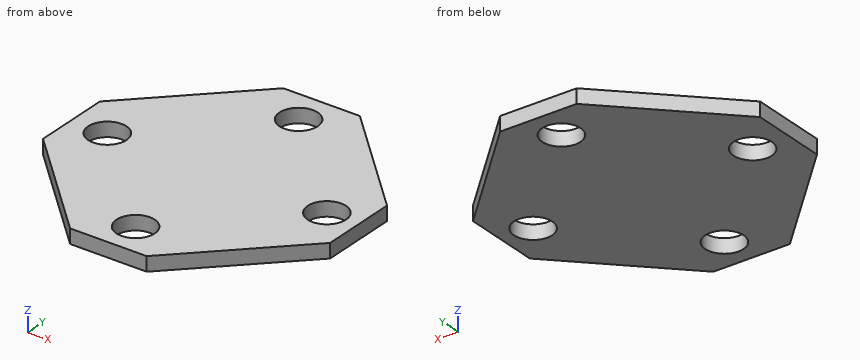
from build123d import *

# Parameters (mm, degrees)
BOSS_EXTRUDE2_DEPTH = 3
SKETCH1_3_R         = 4
CUT_EXTRUDE1_DEPTH  = 4
CIRPATTERN4_COUNT   = 4


with BuildPart() as part:
    # Sketch1 → Boss-Extrude2 (new body)
    with BuildSketch(Plane.XY):
        Polygon((-8, 30), (-30, 8), (-30, -8), (-8, -30), (8, -30), (30, -8), (30, 8), (8, 30), align=None)
    extrude(amount=BOSS_EXTRUDE2_DEPTH)

    # Sketch1<3> → Cut-Extrude1 (cut, through all)
    with BuildSketch(Plane.XY):
        with Locations((-22.5, 0)):
            Circle(SKETCH1_3_R)
    cut_extrude1 = extrude(amount=CUT_EXTRUDE1_DEPTH, mode=Mode.SUBTRACT)

    # CirPattern4: Cut-Extrude1 ×4 about axis
    cirpattern4_axis = Axis((0.438067256, 0, 0), (0, 0, 1))
    for i in range(1, CIRPATTERN4_COUNT):
        add(cut_extrude1.rotate(cirpattern4_axis, i * 360 / CIRPATTERN4_COUNT), mode=Mode.SUBTRACT)


solid = part.part
The listing builds one solid part. Answer for the finished solid, in the listing's coordinates (mm). Round coordinates to 2 decimals unless told otherwise and drop trailing zeros. Write each loop counter-clockwise with the first axis right and the second up, starting at its lowest first coordinate (ties: lowest second). Pieces come first, ordered by that corner, then holes. Notation, with made-up numbers: M 14.25,-24.5 L 25.25,-24.5 A20 ccw 25.25,3.5 Z; hole C -39.75,50 d1. An arc over 180 degrees is marked long. Write each question's results on one line, items separated by ' | '. Start each with the question number.
Item 1: A flat-ended cylindrical pin translates along its axis: pin 1 Ø1.5 at (x, z) = (17.5, 0.5) entering from -Y. Find the tip coordinate at first contact, or state that the pin passes through.
Item 2: A cutting plane is placed at B-B on y = 0. Write down the section's boundary in (x, z), and give its area (3 significant figures).
Item 3: A cutting plane is placed at C-C on z = 1.25. Write down the section's boundary in (x, y), and give its area (3 significant figures).
Item 4: Straight lines are drawn through the part: L1, parallel to X at y = 0, z = 2.4; L2, parallel to X at y = 3.5, z = 1.25; L3, parallel to Y at x = 0.5, z = 2.35. For each, find the intervals that lie inside material, in ascending order. Write a range as [from, to].
Item 5: A cutting plane is placed at D-D on x = 3. Write down the section's boundary in (y, z), and give its area (3 significant figures).
Item 6: A cutting plane is placed at A-A on x = -22.5. Write down the section's boundary in (y, z).
Check sheet entries:
1) pin 1: y = -21.25
2) outline: M -30,0 L -26.5,0 L -26.5,3 L -30,3 Z; M -18.5,0 L 19.38,0 L 19.38,3 L -18.5,3 Z; M 27.38,0 L 30,0 L 30,3 L 27.38,3 Z | area: 132 mm²
3) outline: M -30,-8 L -8,-30 L 8,-30 L 30,-8 L 30,8 L 8,30 L -8,30 L -30,8 Z; hole C -22.5,0 d8; hole C 0.44,-22.94 d8; hole C 0.44,22.94 d8; hole C 23.38,0 d8 | area: 2,430 mm²
4) L1: [-30, -26.5], [-18.5, 19.38], [27.38, 30] | L2: [-30, -24.44], [-20.56, 21.44], [25.31, 30] | L3: [-30, -26.94], [-18.94, 18.94], [26.94, 30]
5) outline: M -30,0 L -26.01,0 L -26.01,3 L -30,3 Z; M -19.87,0 L 19.87,0 L 19.87,3 L -19.87,3 Z; M 26.01,0 L 30,0 L 30,3 L 26.01,3 Z | area: 143 mm²
6) outline: M -15.5,0 L -4,0 L -4,3 L -15.5,3 Z; M 4,0 L 15.5,0 L 15.5,3 L 4,3 Z
